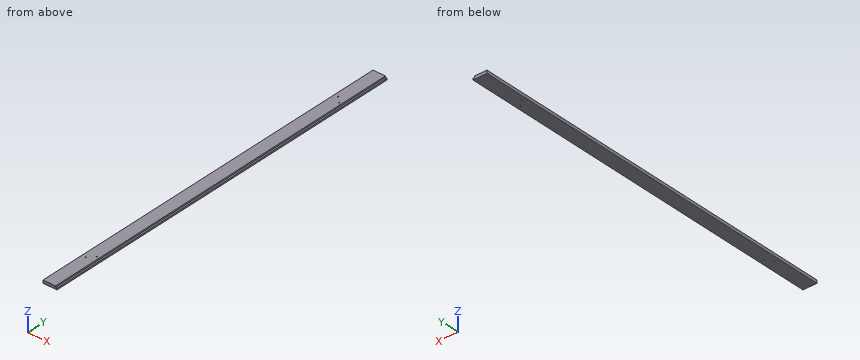
from build123d import *

# Parameters (mm, degrees)
F0_W     = 88.9
F0_H     = 19.05
F1_DEPTH = 1219.2
F2_W     = 44.1598849037
F2_H     = 21.9993637201
F3_DEPTH = 2438.401
F5_R     = 3.175
F6_DEPTH = 19.05


with BuildPart() as f1:
    # F0 (on Front) → F1 (new body, symmetric)
    with BuildSketch(Plane.XZ):
        Rectangle(F0_W, F0_H)
    extrude(amount=F1_DEPTH, both=True)

    # F2 (on face) → F3 (cut, through all)
    with BuildSketch(Plane.XZ.offset(1219.2)):
        with Locations((57.0049424518, 10.9996818601)):
            Rectangle(F2_W, F2_H)
    extrude(amount=-F3_DEPTH, mode=Mode.SUBTRACT)

    # F5 (on face) → F6 (cut, through all)
    with BuildSketch(Plane.XY.offset(9.525)):
        with Locations((19.05, -895.35)):
            Circle(F5_R)
        with Locations((-19.05, -933.45)):
            Circle(F5_R)
        with Locations((-19.05, 933.45)):
            Circle(F5_R)
        with Locations((19.05, 895.35)):
            Circle(F5_R)
    extrude(amount=-F6_DEPTH, mode=Mode.SUBTRACT)


solid = f1.part
Geometry: final body of the model. Coordinates: model frame, mm. Give positions to 0.01 mm unless a question says otherwise; leave off trailing zeros. Write each loop counter-clockwise with the first axis right and the second up, starting at its lowest first coordinate (ties: lowest second). Pieces come first, ordered by that corner, then holes. Notation, with made-up numbers: (29, 73.25) -> (55, 73.25) arc R11 ccw to (55, 89.25) -> close; hole circle Ø1 at (87, 77). An arc over 180 degrees is marked (long way). Answer in a Markdown table with one row per item.
(1) Pin query (flat end, axial travel): pin 1 (5 mm diameter, centred on y = 506, z = 4, fed in from +X) (3 decimals); pin 2 (7.5 mm diameter, centred on x = 40, y = 586.5, fed in from +Z). Return the tip coordinate at first contact, or that it passes through.
Answers below:
| item | result |
|---|---|
| pin 1 | x = 34.925 |
| pin 2 | z = 0 |
(2) Ray query, line 1 along Y through (x, z) = (17.5, 8.5); line 2 along Y through (x, z) = (19.05, -5) (3 decimals); line 3 along X through (y, z) = (895.35, 0.25) (3 decimals). Return the intervals inside material, ascending. Write a range as [from, to].
Answers below:
| item | result |
|---|---|
| line 1 | [-1219.2, -898.12], [-892.58, 892.58], [898.12, 1219.2] |
| line 2 | [-1219.2, -898.525], [-892.175, 892.175], [898.525, 1219.2] |
| line 3 | [-44.45, 15.875], [22.225, 34.925] |
(3) Section query A-A on z = 6.5. Return loops of the section in (x, y) (3 decimals), then the cut area to 3 significant figures.
Answers below:
| item | result |
|---|---|
| outline | (-44.45, -1219.2) -> (34.925, -1219.2) -> (34.925, 1219.2) -> (-44.45, 1219.2) -> close; hole circle Ø6.35 at (-19.05, -933.45); hole circle Ø6.35 at (-19.05, 933.45); hole circle Ø6.35 at (19.05, -895.35); hole circle Ø6.35 at (19.05, 895.35) |
| area | 193,000 mm^2 |
(4) Section query B-B on y = 362. Return loops of the section in (x, z) (3 decimals).
Answers below:
| item | result |
|---|---|
| outline | (-44.45, -9.525) -> (44.45, -9.525) -> (44.45, 0) -> (34.925, 0) -> (34.925, 9.525) -> (-44.45, 9.525) -> close |
